from build123d import *

# Parameters (mm, degrees)
IZIM2_R               = 20
KES_EKSTR_ZYON1_DEPTH = 160
IZIM3_R               = 25
KES_EKSTR_ZYON2_DEPTH = 120
KES_EKSTR_ZYON3_DEPTH = 120


with BuildPart() as part:
    # Çizim1 → Döndür1 (revolve)
    with BuildSketch(Plane(origin=(0, 0, 379.673045167), x_dir=(-1, 0, 0), z_dir=(0, 0, -1)), mode=Mode.PRIVATE) as d_nd_r1_sk:
        Polygon((-2016.208991354, 150), (-2016.208991354, 0), (-1934.353602541, 0), (-1934.353602541, 150), (-1940.492756702, 150), (-1948.000467843, 125.443383356), (-1961.634431646, 125.443383356), (-1969.142142787, 150), (-1981.420451109, 150), (-1988.928162249, 125.443383356), (-2002.562126052, 125.443383356), (-2010.069837193, 150), align=None)
    revolve(d_nd_r1_sk.sketch.rotate(Axis((2016.208991354, 0, 379.673045167), (-1, 0, 0)), 270), axis=Axis((2016.208991354, 0, 379.673045167), (-1, 0, 0)))

    # Çizim2 → Kes-Ekstrüzyon1 (cut)
    with BuildSketch(Plane.ZY.offset(-1934.353602541)):
        with Locations((379.673045167, 0)):
            Circle(IZIM2_R)
    extrude(amount=-KES_EKSTR_ZYON1_DEPTH, mode=Mode.SUBTRACT)

    # Çizim3 → Kes-Ekstrüzyon2 (cut)
    with BuildSketch(Plane(origin=(2016.208991354, 0, 0), x_dir=(0, 0, -1), z_dir=(1, 0, 0))):
        with Locations((-379.673045167, 0)):
            Circle(IZIM3_R)
    extrude(amount=-KES_EKSTR_ZYON2_DEPTH, mode=Mode.SUBTRACT)

    # Çizim4 → Kes-Ekstrüzyon3 (cut)
    with BuildSketch(Plane(origin=(2016.208991354, 0, 0), x_dir=(0, 0, -1), z_dir=(1, 0, 0))):
        with BuildLine():
            Line((-379.673045167, 29), (-379.673045167, 25))
            ThreePointArc((-379.673045167, 25), (-377.666572387, 24.919351255), (-375.673045167, 24.677925359))
            Line((-375.673045167, 24.677925359), (-375.673045167, 29))
            Line((-375.673045167, 29), (-379.673045167, 29))
        make_face()
        with BuildLine():
            ThreePointArc((-383.673045167, 24.677925359), (-381.679517947, 24.919351255), (-379.673045167, 25))
            Line((-379.673045167, 25), (-379.673045167, 29))
            Line((-379.673045167, 29), (-383.673045167, 29))
            Line((-383.673045167, 29), (-383.673045167, 24.677925359))
        make_face()
    extrude(amount=-KES_EKSTR_ZYON3_DEPTH, mode=Mode.SUBTRACT)


solid = part.part
The model under review builds one solid part; all positions refer to its coordinate system, in mm. A direction names the side the tool comes from. Coordinates: 2 decimals unless noted, no trailing zeros. Write each loop counter-clockwise with the first axis right and the second up, starting at its lowest first coordinate (ties: lowest second). Pieces come first, ordered by that corner, then holes. Notation, with made-up numbers: (60, -17.5) - (115, -17.5) arc R17 ccw to (115, -13.5) - close; hole circle Ø7 at (0.25, 3). An arc over 180 degrees is marked (long way). Answer as a JSON object with one key per item and string values. Group by question number.
1. Add section B-B (x = 1944). Give the boundary of the cut face in (y, z).
2. Mouldability with a two-part tool opening along X and no side actions: class faces 1 (the face through (1995.841, 84.781, 287.216)), 2 (the face through (1934.354, 2, 348)), 3 (the face through (1975.85, -24.98, 380.72)), 4 (the face through (1988.564, 5.568, 253.16)) as pulls with the +X half, pulls with the -X half, needs draft (parallel to the pull), parting line crosses it, or undercut.
3. Add section A-A (y = 0). Give the boundary of the cut face in (x, z).
4. Machinability: for faces 5 (the face through (2003.03, -48.63, 496.97)), 6 (the face through (1976, 29, 380)), 7 (the face through (2016.209, 2, 411)), which of the approach directions +Z, -Z, +X, -X, +Y, -Y give a long, thin tool a straight path to every point of the face, cutting with its end or side? Answer none if there is none.
5. To check wall thickness, follow probe 1 along Y at (x, z) = (1950, 380); probe 2 along X at (y, z) = (137, 425); probe 3 along Y at (x, z) = (1998, 399). State the ranges of each line that lie inside material, in increasing order.
6. Clearance check with flat-ended pins moving along their axes: pin 1 Ø8 at (x, y) = (1976.5, -61) entering from +Z; pin 2 Ø5 at (x, y) = (1957, 27.5) entering from +Z; pin 3 Ø4 at (x, z) = (1998.5, 366.5) entering from +Y. State where each tip first meets the part, or that it passes through.
Findings:
{
 "1": {"outline": "circle Ø277.06 at (0, 379.67); hole (24.68, 375.67) - (29, 375.67) - (29, 383.67) - (24.68, 383.67) arc R25 ccw (long way) to start"},
 "2": {"face 1": "undercut", "face 2": "pulls with the -X half", "face 3": "needs draft", "face 4": "undercut"},
 "3": {"outline": "(1934.35, 229.67) - (1940.49, 229.67) - (1948, 254.23) - (1961.63, 254.23) - (1969.14, 229.67) - (1981.42, 229.67) - (1988.93, 254.23) - (2002.56, 254.23) - (2010.07, 229.67) - (2016.21, 229.67) - (2016.21, 354.67) - (1934.35, 354.67) - close; (1934.35, 404.67) - (2016.21, 404.67) - (2016.21, 529.67) - (2010.07, 529.67) - (2002.56, 505.12) - (1988.93, 505.12) - (1981.42, 529.67) - (1969.14, 529.67) - (1961.63, 505.12) - (1948, 505.12) - (1940.49, 529.67) - (1934.35, 529.67) - close"},
 "4": {"face 5": "none", "face 6": "+X, -X", "face 7": "+Z, -Z, +X, +Y, -Y"},
 "5": {"probe 1": "-125.44 to -25, 29 to 125.44", "probe 2": "1934.35 to 1942.23, 1967.4 to 1983.16, 2008.33 to 2016.21", "probe 3": "-123.95 to -15.86, 15.86 to 123.95"},
 "6": {"pin 1": "z = 518.42", "pin 2": "z = 502.6", "pin 3": "y = 124.94"}
}
